The listing builds one solid part. Answer for the finished solid, in the listing's coordinates (mm). Face numbers are marked on the shaded views. Coordinates: 2 decimals unless noted, no trailing zeros. Order: outer loops, then holes, each group sorted by start corner. A loop starts at its lowest first (then second) coordinate and runs counter-clockwise, first axis right, second up. Notation, with made-up numbers: (89.5, 57.25) - (138.5, 57.25) arc R26 ccw to (138.5, 95.25) - close; hole circle Ø6 at (2, 33). An arc over 180 degrees is marked (long way). Use a Markdown table: item, result. Add a question column.
Item 1: The part is cut by section A-A, the plane x = -51.5. Give the vertices of the cut face in (y, z).
Item 2: The mould has two halves that part along X. Classify the marked faces 1, 2 and 3: released by +X, released by -X, zero draft, split by the parting line, or undercut.
Item 3: The part is cut by section C-C, the plane y = 40.5. Give the vertices of the cut face in (x, z).
Item 4: The part is cut by section D-D, the plane x = -24. Give the vertices of the cut face in (y, z).
Item 5: The part is cut by section B-B, the plane z = -65. Give the vertices of the cut face in (x, y).
Item 6: Find the intervals of material crossed by line 1 along Y through (x, z) = (-102.8, -4); line 2 along X through (y, z) = (-9, -20.5); line 3 along Z through (x, y) = (95.5, 13.5), in increasing order.
Item 7: Flat-ended cylindrical pins translate along their axes: P1, Ø2.5, axis at y = 56, z = -2.5, coming from the +X side; P2, Ø3, axis at y = -59.5, z = -38.5, coming from the +X side; P3, Ø0.9, axis at x = 103, y = 3, coming from the -Z side; P4, Ø1.5, axis at y = 50.5, z = -6.5, coming from the +X side. Find the tip coordinate at first contact, or state that the pin passes through.
from build123d import *

# Parameters (mm, degrees)
BOSS_EXTRUDE1_DEPTH     = 3
SKETCH1_3_W             = 70
SKETCH1_3_H             = 176
SKETCH1_3_W_2           = 66
SKETCH1_3_H_2           = 172
BOSS_EXTRUDE2_DEPTH     = 5
SKETCH1_4_W             = 66
SKETCH1_4_H             = 25
BOSS_EXTRUDE3_DEPTH     = 25
CUT_EXTRUDE1_START      = -3
SKETCH2_R               = 12.5
SKETCH2_R_2             = 1.5
CUT_EXTRUDE1_DEPTH      = 202.50659462
SKETCH2_4_R             = 1.5
SKETCH2_4_R_2           = 4
CUT_EXTRUDE2_DEPTH      = 1
CUT_EXTRUDE2_DEPTH_BACK = 209.50659462
SKETCH5_R               = 14.5
CUT_EXTRUDE3_DEPTH      = 15.5
SKETCH6_W               = 4
SKETCH6_H               = 55
BOSS_EXTRUDE4_DEPTH     = 70
SKETCH7_R               = 1.6
CUT_EXTRUDE4_DEPTH      = 4


with BuildPart() as part:
    # Sketch1 → Boss-Extrude1 (new body)
    with BuildSketch(Plane.XY):
        with BuildLine():
            ThreePointArc((104.25329731, 12.5), (0, 105), (-104.25329731, 12.5))
            Line((-104.25329731, 12.5), (-104.25329731, -12.5))
            ThreePointArc((-104.25329731, -12.5), (0, -105), (104.25329731, -12.5))
            Line((104.25329731, -12.5), (104.25329731, 12.5))
        make_face()
    extrude(amount=BOSS_EXTRUDE1_DEPTH)

    # Sketch1_3 → Boss-Extrude2 (add)
    with BuildSketch(Plane.XY):
        Rectangle(SKETCH1_3_W, SKETCH1_3_H)
        Rectangle(SKETCH1_3_W_2, SKETCH1_3_H_2, mode=Mode.SUBTRACT)
    extrude(amount=-BOSS_EXTRUDE2_DEPTH)

    # Sketch1_4 → Boss-Extrude3 (add)
    with BuildSketch(Plane.XY):
        with Locations((-71.25329731, 0)):
            Rectangle(SKETCH1_4_W, SKETCH1_4_H)
        with Locations((71.25329731, 0)):
            Rectangle(SKETCH1_4_W, SKETCH1_4_H)
    extrude(amount=-BOSS_EXTRUDE3_DEPTH)

    # Sketch2 → Cut-Extrude1 (cut)
    with BuildSketch(Plane.ZY.offset(104.25329731).offset(CUT_EXTRUDE1_START)):
        with Locations((-12.5, 0)):
            Circle(SKETCH2_R)
        with Locations((-4, 0)):
            Circle(SKETCH2_R_2, mode=Mode.SUBTRACT)
        with Locations((-21, 0)):
            Circle(SKETCH2_R_2, mode=Mode.SUBTRACT)
        with BuildLine():
            ThreePointArc((-25, 2.5e-08), (-21.338834756, 8.838834774), (-12.5, 12.5))
            Line((-12.5, 12.5), (-25, 12.5))
            Line((-25, 12.5), (-25, 2.5e-08))
        make_face()
        with BuildLine():
            ThreePointArc((-12.5, -12.5), (-21.338834774, -8.838834756), (-25, 2.5e-08))
            Line((-25, 2.5e-08), (-25, -12.5))
            Line((-25, -12.5), (-12.5, -12.5))
        make_face()
    extrude(amount=-CUT_EXTRUDE1_DEPTH, mode=Mode.SUBTRACT)


with BuildPart() as cut_extrude1_piece_1:
    # of the 3 separate pieces the step leaves, piece 1, a body of its own (cut_extrude1_pieces)
    add(part.part.solids().sort_by_distance((104.25329731, -12.5, 0))[0])


with BuildPart() as cut_extrude1_piece_2:
    # of the 3 separate pieces the step leaves, piece 2, a body of its own (cut_extrude1_pieces)
    add(part.part.solids().sort_by_distance((-35, -1.118033989, -5))[0])


with BuildPart() as cut_extrude1_piece_3:
    # of the 3 separate pieces the step leaves, piece 3, a body of its own (cut_extrude1_pieces)
    add(part.part.solids().sort_by_distance((35, 1.118033989, -5))[0])


with BuildPart() as cut_extrude2_tool:
    # Sketch2_4 → Cut-Extrude2 (new, two sides)
    with BuildSketch(Plane.ZY.offset(104.25329731)) as cut_extrude2_sk:
        with Locations((-21, 0)):
            Circle(SKETCH2_4_R)
        with Locations((-4, 0)):
            Circle(SKETCH2_4_R)
        with Locations((-12.5, 0)):
            Circle(SKETCH2_4_R_2)
    extrude(amount=CUT_EXTRUDE2_DEPTH)
    extrude(cut_extrude2_sk.sketch, amount=-CUT_EXTRUDE2_DEPTH_BACK)


with BuildPart() as cut_extrude1_piece_1_1:
    add(cut_extrude1_piece_1.part)

    # Cut-Extrude2: cut by cut_extrude2_tool
    add(cut_extrude2_tool.part, mode=Mode.SUBTRACT)

    # Sketch4 one side → Revolve1 (revolve)
    with BuildSketch(Plane(origin=(0, 0, 0), x_dir=(0, 0, -1), z_dir=(1, 0, 0))):
        with BuildLine():
            Line((-17.5, 90.5), (-3, 90.5))
            Line((-3, 90.5), (-3, 105))
            ThreePointArc((-3, 105), (-13.253048327, 100.753048327), (-17.5, 90.5))
        make_face()
    revolve(axis=Axis((0, 90.5, 17.5), (0, 0, -1)))

    # Sketch4_4 one side → Revolve2 (revolve)
    with BuildSketch(Plane(origin=(0, 0, 0), x_dir=(0, 0, -1), z_dir=(1, 0, 0))):
        with BuildLine():
            Line((-17.5, -90.5), (-3, -90.5))
            Line((-3, -90.5), (-3, -76))
            ThreePointArc((-3, -76), (-13.253048327, -80.246951673), (-17.5, -90.5))
        make_face()
    revolve(axis=Axis((0, -90.5, 17.5), (0, 0, -1)))

    # Sketch5 → Cut-Extrude3 (cut, through all)
    with BuildSketch(Plane.XY.offset(3)):
        with Locations((0, -90.5)):
            Circle(SKETCH5_R)
        with Locations((0, 90.5)):
            Circle(SKETCH5_R)
    extrude(amount=CUT_EXTRUDE3_DEPTH, mode=Mode.SUBTRACT)

    # Sketch6 → Boss-Extrude4 (add)
    with BuildSketch(Plane(origin=(0, 0, 0), x_dir=(-1, 0, 0), z_dir=(0, 0, -1))):
        with Locations((-75, -42)):
            Rectangle(SKETCH6_W, SKETCH6_H)
    extrude(amount=BOSS_EXTRUDE4_DEPTH)

    # Sketch7 → Cut-Extrude4 (cut)
    with BuildSketch(Plane(origin=(77, 0, 0), x_dir=(0, 0, -1), z_dir=(1, 0, 0))):
        with Locations((2.54, -33.09)):
            Circle(SKETCH7_R)
        with Locations((54.61, -66.13)):
            Circle(SKETCH7_R)
    extrude(amount=-CUT_EXTRUDE4_DEPTH, mode=Mode.SUBTRACT)


with BuildPart() as cut_extrude1_piece_2_1:
    add(cut_extrude1_piece_2.part)

    # Cut-Extrude2: cut by cut_extrude2_tool
    add(cut_extrude2_tool.part, mode=Mode.SUBTRACT)


with BuildPart() as cut_extrude1_piece_3_1:
    add(cut_extrude1_piece_3.part)

    # Cut-Extrude2: cut by cut_extrude2_tool
    add(cut_extrude2_tool.part, mode=Mode.SUBTRACT)


solid = cut_extrude1_piece_1_1.part
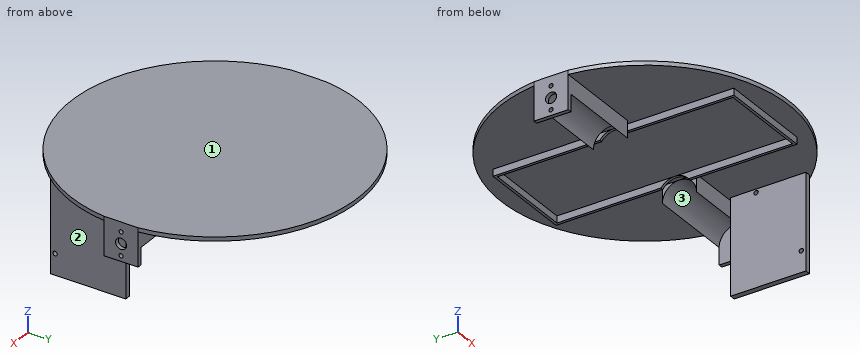
Solution:
| question | item | result |
|---|---|---|
| 1 | outline | (-91.5, 0) - (-12.5, 0) - (-12.5, -12.5) arc R12.5 cw to (12.5, -12.5) - (12.5, 0) - (91.5, 0) - (91.5, 3) - (-91.5, 3) - close |
| 2 | face 1 | zero draft |
| 2 | face 2 | released by +X |
| 2 | face 3 | undercut |
| 3 | outline | (-96.87, 0) - (-35, 0) - (-35, -5) - (-33, -5) - (-33, 0) - (33, 0) - (33, -5) - (35, -5) - (35, 0) - (96.87, 0) - (96.87, 3) - (-96.87, 3) - close |
| 4 | outline | (-102.22, 0) - (-88, 0) - (-88, -5) - (-86, -5) - (-86, 0) - (86, 0) - (86, -5) - (88, -5) - (88, 0) - (102.22, 0) - (102.22, 3) - (-102.22, 3) - close |
| 5 | outline | (73, -69.5) - (77, -69.5) - (77, -14.5) - (73, -14.5) - close |
| 6 | line 1 | y = -12.5 to -1.5, 1.5 to 12.5 |
| 6 | line 2 | x = -104.25 to -101.25, 101.25 to 104.25 |
| 6 | line 3 | z = 0 to 3 |
| 7 | P1 | stops at x = 35 |
| 7 | P2 | stops at x = 77 |
| 7 | P3 | stops at z = -25 |
| 7 | P4 | passes through |
